Geometry check sheet. Reference: the model listing, model coordinates, mm. A direction names the side the tool comes from. Coordinates: 2 decimals unless noted, no trailing zeros. Write each loop counter-clockwise with the first axis right and the second up, starting at its lowest first coordinate (ties: lowest second). Pieces come first, ordered by that corner, then holes. Notation, with made-up numbers: (8.5, -30.5) -> (54.5, -30.5) arc R17 ccw to (54.5, -20.5) -> close; hole circle Ø1 at (-15.75, -20.5). An arc over 180 degrees is marked (long way). Answer in a Markdown table with one row per item. Add a question column.
1. Scan lines: L1, parallel to Y at x = -209, z = -0.85; L2, parallel to Y at x = -210.5, z = -0.45. Record each from-to range of solid material in increasing order. Write a range as from..to.
2. Cross-section at B-B on x = -207. Record the cut outline in (y, z), and give its area (3 significant figures).
3. Cross-section at C-C on z = -0.8. Record the cut outline in (x, y).
4. Cross-section at A-A on y = 68.4. Record the cut outline in (x, z), and give its area (3 significant figures).
5. Set-up check for faces 1 (the flat face through (-212.9, 68.7, -0.35)), 2 (the flat face through (-213, 68.5, -0.65)): record each of +Z, -Z, +X, -X, +Y, -Y from which the full face is reachable in a straight line by a thin tool's end or side.
```python
from build123d import *

# Parameters (mm, degrees)
BOX111_W               = 0.8
BOX111_H               = 17
BOX111_DEPTH           = 0.8
BOX112_W               = 0.8
BOX112_H               = 14
BOX112_DEPTH           = 0.8
CUT059_PLACEMENT_ANGLE = 72


with BuildPart() as cubo111:
    # Box111 → Box111 (new body)
    with BuildSketch(Plane.XY):
        with Locations((0.4, 8.5)):
            Rectangle(BOX111_W, BOX111_H)
    extrude(amount=BOX111_DEPTH)


with BuildPart() as obj1:
    # Box112 → Box112 (new body)
    with BuildSketch(Plane(origin=(0.3, 0, 0.3), x_dir=(1, 0, 0), z_dir=(0, 0, 1))):
        with Locations((0.4, 7)):
            Rectangle(BOX112_W, BOX112_H)
    extrude(amount=BOX112_DEPTH)

    # Cut059: cut Cubo111
    add(cubo111.part, mode=Mode.SUBTRACT)


with BuildPart() as obj1_1:
    # Cut059 placement: moved
    add(obj1.part.moved(Location((-206.4, 65.8, -1.45))).rotate(Axis((-206.4, 65.8, -1.45), (0, 0, 1)), CUT059_PLACEMENT_ANGLE))


solid = obj1_1.part
```
Results found:
| question | item | result |
|---|---|---|
| 1 | L1 | y = 67.49..67.8 |
| 1 | L2 | y = 67.45..68.29 |
| 2 | outline | (66.31, -0.65) -> (66.84, -0.65) -> (66.84, -1.15) -> (67.15, -1.15) -> (67.15, -0.35) -> (66.31, -0.35) -> close |
| 2 | area | 0.410 mm^2 |
| 3 | outline | (-219.47, 70.89) -> (-206.15, 66.56) -> (-206.06, 66.85) -> (-219.37, 71.17) -> close |
| 4 | outline | (-213.43, -0.65) -> (-211.81, -0.65) -> (-211.81, -1.15) -> (-210.84, -1.15) -> (-210.84, -0.35) -> (-213.43, -0.35) -> close |
| 4 | area | 1.26 mm^2 |
| 5 | face 1 | +Z, +X, -X, +Y, -Y |
| 5 | face 2 | -Z, -X, -Y |
